```python
from build123d import *

# Parameters (mm, degrees)
SKETCH1_W               = 198
SKETCH1_H               = 90
BOSS_EXTRUDE1_DEPTH     = 4
SKETCH3_R               = 2
CUT_EXTRUDE1_DEPTH      = 10
SKETCH4_R               = 1
BOSS_EXTRUDE3_DEPTH     = 24
BOSS_EXTRUDE4_DEPTH     = 25
CUT_EXTRUDE2_DEPTH      = 219.926928449
CUT_EXTRUDE2_DEPTH_BACK = 219.926928449
SKETCH4_5_R             = 1


with BuildPart() as part:
    # Sketch1 → Boss-Extrude1 (new body)
    with BuildSketch(Plane.XY):
        with Locations((99, 45)):
            Rectangle(SKETCH1_W, SKETCH1_H)
    extrude(amount=BOSS_EXTRUDE1_DEPTH)

    # Sketch3 → Cut-Extrude1 (cut)
    with BuildSketch(Plane(origin=(0, 0, 0), x_dir=(-1, 0, 0), z_dir=(0, 0, -1))):
        with Locations((-191, 20)):
            Circle(SKETCH3_R)
        with Locations((-191, 70)):
            Circle(SKETCH3_R)
        with Locations((-7, 20)):
            Circle(SKETCH3_R)
        with Locations((-7, 70)):
            Circle(SKETCH3_R)
    extrude(amount=-CUT_EXTRUDE1_DEPTH, mode=Mode.SUBTRACT)

    # Sketch4 → Boss-Extrude3 (add)
    # profile 1 of 6: a face of its own
    with BuildSketch(Plane.XY.offset(4)):
        Polygon((13.8, 88.01600051), (13.8, 79.750184794), (15.052652573, 79.750184794), (21.052652573, 79.750184794), (21.052652573, 85.750184794), (21.052652573, 88.01600051), align=None)
        with Locations((18.052652573, 82.750184794)):
            Circle(SKETCH4_R, mode=Mode.SUBTRACT)
    # profile 2 of 6: a face of its own
    with BuildSketch(Plane.XY.offset(4)):
        Polygon((21.052652573, 35.092027634), (15.052652573, 35.092027634), (13.8, 35.092027634), (13.8, 25.580021251), (21.052652573, 25.580021251), (21.052652573, 28.314099722), align=None)
        with Locations((18.052652573, 32.092027634)):
            Circle(SKETCH4_R, mode=Mode.SUBTRACT)
    # profile 3 of 6: a face of its own
    with BuildSketch(Plane.XY.offset(4)):
        Polygon((84.2, 35.092027634), (82.855604308, 35.092027634), (76.855604308, 35.092027634), (76.855604308, 29.092027634), (76.855604308, 25.580021251), (84.2, 25.580021251), align=None)
        with Locations((79.855604308, 32.092027634)):
            Circle(SKETCH4_R, mode=Mode.SUBTRACT)
    # profile 4 of 6: a face of its own
    with BuildSketch(Plane.XY.offset(4)):
        with Locations((18.052652573, 32.092027634)):
            Circle(SKETCH4_R)
    # profile 5 of 6: a face of its own
    with BuildSketch(Plane.XY.offset(4)):
        with Locations((18.052652573, 82.750184794)):
            Circle(SKETCH4_R)
    # profile 6 of 6: a face of its own
    with BuildSketch(Plane.XY.offset(4)):
        with Locations((79.855604308, 32.092027634)):
            Circle(SKETCH4_R)
    extrude(amount=BOSS_EXTRUDE3_DEPTH)

    # Sketch4_4 → Boss-Extrude4 (add)
    with BuildSketch(Plane.XY.offset(4)):
        Polygon((13, 79.750184794), (13.8, 79.750184794), (13.8, 88.01600051), (21.052652573, 88.01600051), (21.052652573, 88.5), (13, 88.5), align=None)
        Polygon((13.8, 25.580021251), (13.8, 35.092027634), (13, 35.092027634), (13, 24.280021251), (21.052652573, 24.280021251), (21.052652573, 25.580021251), align=None)
        Polygon((85.5, 35.092027634), (84.2, 35.092027634), (84.2, 25.580021251), (76.855604308, 25.580021251), (76.855604308, 24.280021251), (85.5, 24.280021251), align=None)
    extrude(amount=BOSS_EXTRUDE4_DEPTH)

    # Sketch4_5 → Cut-Extrude2 (cut, two sides: drawn at the far end of the back side and taken through both)
    with BuildSketch(Plane.XY.offset(4).offset(-CUT_EXTRUDE2_DEPTH_BACK)):
        with Locations((18.052652573, 82.750184794)):
            Circle(SKETCH4_5_R)
        with Locations((18.052652573, 32.092027634)):
            Circle(SKETCH4_5_R)
        with Locations((79.855604308, 32.092027634)):
            Circle(SKETCH4_5_R)
    extrude(amount=CUT_EXTRUDE2_DEPTH + CUT_EXTRUDE2_DEPTH_BACK, mode=Mode.SUBTRACT)


solid = part.part
```
Could you check a few things on this model? Use its own coordinates, in mm. A direction names the side the tool comes from. Round coordinates to 2 decimals unless told otherwise and drop trailing zeros. Loops run counter-clockwise (first coordinate to the right, second up) from the corner with the lowest first, then second, coordinate; pieces in that order, holes last. Notation, with made-up numbers: (32, -27.75) - (55, -27.75) arc R17 ccw to (55, -2.75) - close; hole circle Ø8 at (48, 8.25). An arc over 180 degrees is marked (long way). Answer in a Markdown table with one row per item. Add a question column.
(1) If we section it at D-D (x = 147): Please give me the cut outline in (y, z).
(2) If we section it at B-B (y = 20): Please give me the cut outline in (x, z).
(3) I need wall thicknesses on line 1 along Y through (x, z) = (7, 2.4); line 2 along X through (y, z) = (25.5, 22); line 3 along Z through (x, y) = (93, 12). Which ranges of each line are inside material? Lowest first, please.
(4) If we mould it in two halves opening along Y, with no side actions, what happens to faces 6 (the face through (17, 79.75, 16)), 7 (the face through (17, 24.28, 16)), 8 (the face through (13.4, 27.3, 29))? For each: pulls with the +Y half, pulls with the -Y half, needs draft (parallel to the pull), parting line crosses it, or undercut.
(5) For faces 1 (the face through (21.053, 84, 16)), 2 (the face through (76.856, 30, 16)), 3 (the face through (81, 24.28, 16)), 4 (the face through (13, 84, 16)), 5 (the face through (17, 88.5, 16)), which set-ups out of +Z, -Z, +X, -X, +Y, -Y let a thin tool reach every point of the face, with its end or its side?
(6) If we section it at A-A (x = 7): Please give me the cut outline in (y, z), plus the area to 3 significant figures.
(7) I'm going to push flat-ended pins straight in: pin 1 (0.5 mm diameter, centred on y = 28, z = 28.5, fed in from -X); pin 2 (4.5 mm diameter, centred on x = 81.5, z = 15, fed in from -Y); pin 3 (6 mm diameter, centred on x = 157.5, y = 54, fed in from +Z); pin 4 (6 mm diameter, centred on x = 18.5, y = 86, fed in from +Z). Where does each tip first touch, or does it pass through?
(8) If we section it at C-C (z = 20.5): Please give me the cut outline in (x, y).
Model answer:
| question | item | result |
|---|---|---|
| 1 | outline | (0, 0) - (90, 0) - (90, 4) - (0, 4) - close |
| 2 | outline | (0, 0) - (5, 0) - (5, 4) - (0, 4) - close; (9, 0) - (189, 0) - (189, 4) - (9, 4) - close; (193, 0) - (198, 0) - (198, 4) - (193, 4) - close |
| 3 | line 1 | y = 0 to 18, 22 to 68, 72 to 90 |
| 3 | line 2 | x = 13 to 21.05, 76.86 to 85.5 |
| 3 | line 3 | z = 0 to 4 |
| 4 | face 6 | undercut |
| 4 | face 7 | pulls with the -Y half |
| 4 | face 8 | needs draft |
| 5 | face 1 | +Z, +X, +Y, -Y |
| 5 | face 2 | +Z, +Y, -Y |
| 5 | face 3 | +Z, +X, -X, -Y |
| 5 | face 4 | +Z, -X, +Y, -Y |
| 5 | face 5 | +Z, +X, -X, +Y |
| 6 | outline | (0, 0) - (18, 0) - (18, 4) - (0, 4) - close; (22, 0) - (68, 0) - (68, 4) - (22, 4) - close; (72, 0) - (90, 0) - (90, 4) - (72, 4) - close |
| 6 | area | 328 mm² |
| 7 | pin 1 | stops at x = 13 |
| 7 | pin 2 | stops at y = 24.28 |
| 7 | pin 3 | stops at z = 4 |
| 7 | pin 4 | stops at z = 29 |
| 8 | outline | (13, 24.28) - (21.05, 24.28) - (21.05, 35.09) - (13, 35.09) - close; (13, 79.75) - (21.05, 79.75) - (21.05, 88.5) - (13, 88.5) - close; (76.86, 24.28) - (85.5, 24.28) - (85.5, 35.09) - (76.86, 35.09) - close; hole circle Ø2 at (18.05, 32.09); hole circle Ø2 at (18.05, 82.75); hole circle Ø2 at (79.86, 32.09) |
